from build123d import *

# Parameters (mm, degrees)
CROQUIS1_R              = 1.6
CROQUIS1_R_2            = 1.55
SALIENTE_EXTRUIR1_DEPTH = 3


with BuildPart() as part:
    # Croquis1 → Saliente-Extruir1 (new body)
    with BuildSketch(Plane(origin=(0, 0, 0), x_dir=(1, 0, 0), z_dir=(0, 1, 0))):
        with BuildLine():
            Line((230.847543198, -52.68112687), (230.847543198, 34.350751843))
            ThreePointArc((230.847543198, 34.350751843), (222.131671295, 37.117490889), (214.7720715, 42.544972702))
            Line((214.7720715, 42.544972702), (214.7720715, 0.063564764))
            Line((214.7720715, 0.063564764), (170.847543198, 0.063564764))
            Line((170.847543198, 0.063564764), (170.847543198, 46.193023152))
            Line((170.847543198, 46.193023152), (211.779688747, 46.193023152))
            ThreePointArc((211.779688747, 46.193023152), (208.772718477, 51.86045172), (207.134730277, 58.063564764))
            Line((207.134730277, 58.063564764), (-206.939643881, 58.063564764))
            ThreePointArc((-206.939643881, 58.063564764), (-214.853466929, 42.264574891), (-230.652456802, 34.350751843))
            Line((-230.652456802, 34.350751843), (-230.652456802, -52.936435236))
            Line((-230.652456802, -52.936435236), (-230.652456802, -56.936435236))
            Line((-230.652456802, -56.936435236), (230.847543198, -56.936435236))
            Line((230.847543198, -56.936435236), (230.847543198, -52.68112687))
        make_face()
        with Locations(Location((193.347543198, -3.936435236, 0), (0, 0, 270))):
            Circle(CROQUIS1_R, mode=Mode.SUBTRACT)
        with Locations(Location((193.347543198, 49.063564764, 0), (0, 0, 270))):
            Circle(CROQUIS1_R, mode=Mode.SUBTRACT)
        with Locations(Location((222.847543198, -47.436435236, 0), (0, 0, 270))):
            Circle(CROQUIS1_R_2, mode=Mode.SUBTRACT)
        with Locations(Location((0.097543198, 50.063564764, 0), (0, 0, 270))):
            Circle(CROQUIS1_R, mode=Mode.SUBTRACT)
        with Locations(Location((-222.652456802, -47.436435236, 0), (0, 0, 270))):
            Circle(CROQUIS1_R_2, mode=Mode.SUBTRACT)
    extrude(amount=SALIENTE_EXTRUIR1_DEPTH)


solid = part.part
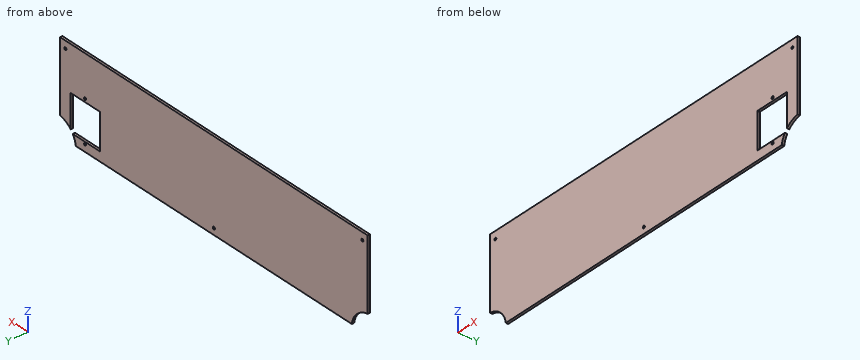
Read the model definition and answer for the solid it produces. Units are mm, in the model's axes. Give positions to 0.01 mm unless a question says otherwise; leave off trailing zeros. Loops run counter-clockwise (first coordinate to the right, second up) from the corner with the lowest first, then second, coordinate; pieces in that order, holes last. Notation, with made-up numbers: (6.25, 75.25) -> (31.25, 75.25) arc R25 cw to (31.25, 92.25) -> close; hole circle Ø1 at (58.25, 62). An arc over 180 degrees is marked (long way). Answer as CSV lines item,"result".
Item 1: Find section A-A on x = 185.5. Give the vertices of the cut face in (y, z), plus the area to 3 significant figures.
Returned:
outline,"(0, -58.06) -> (3, -58.06) -> (3, -46.19) -> (0, -46.19) -> close; (0, -0.06) -> (3, -0.06) -> (3, 56.94) -> (0, 56.94) -> close"
area,"207 mm²"
Item 2: Consider line 1 (X direction, y = 0.35, z = -9); line 2 (Z direction, x = 196.5, y = 2.75); line 3 (X direction, y = 1.35, z = 3.5). Determine where each line is inside the solid, lowest interval first. Write a range as [from, to].
Returned:
line 1,"x = [-230.65, 170.85], [214.77, 230.85]"
line 2,"z = [-58.06, -46.19], [-0.06, 56.94]"
line 3,"x = [-230.65, 191.81], [194.89, 230.85]"
Item 3: Find section C-C on y = 0.5. Give the vertices of the cut face in (x, z), plus the area to 3 significant figures.
Returned:
outline,"(-230.65, -34.35) arc R28 cw to (-206.94, -58.06) -> (207.13, -58.06) arc R28 cw to (211.78, -46.19) -> (170.85, -46.19) -> (170.85, -0.06) -> (214.77, -0.06) -> (214.77, -42.54) arc R28 cw to (230.85, -34.35) -> (230.85, 56.94) -> (-230.65, 56.94) -> close; hole circle Ø3.1 at (-222.65, 47.44); hole circle Ø3.2 at (0.1, -50.06); hole circle Ø3.2 at (193.35, -49.06); hole circle Ø3.2 at (193.35, 3.94); hole circle Ø3.1 at (222.85, 47.44)"
area,"50,200 mm²"
Item 4: Find section B-B on z = -28.5. Give the vertices of the cut face in (x, y).
Returned:
outline,"(-230.65, 0) -> (170.85, 0) -> (170.85, 3) -> (-230.65, 3) -> close; (214.77, 0) -> (230.85, 0) -> (230.85, 3) -> (214.77, 3) -> close"
